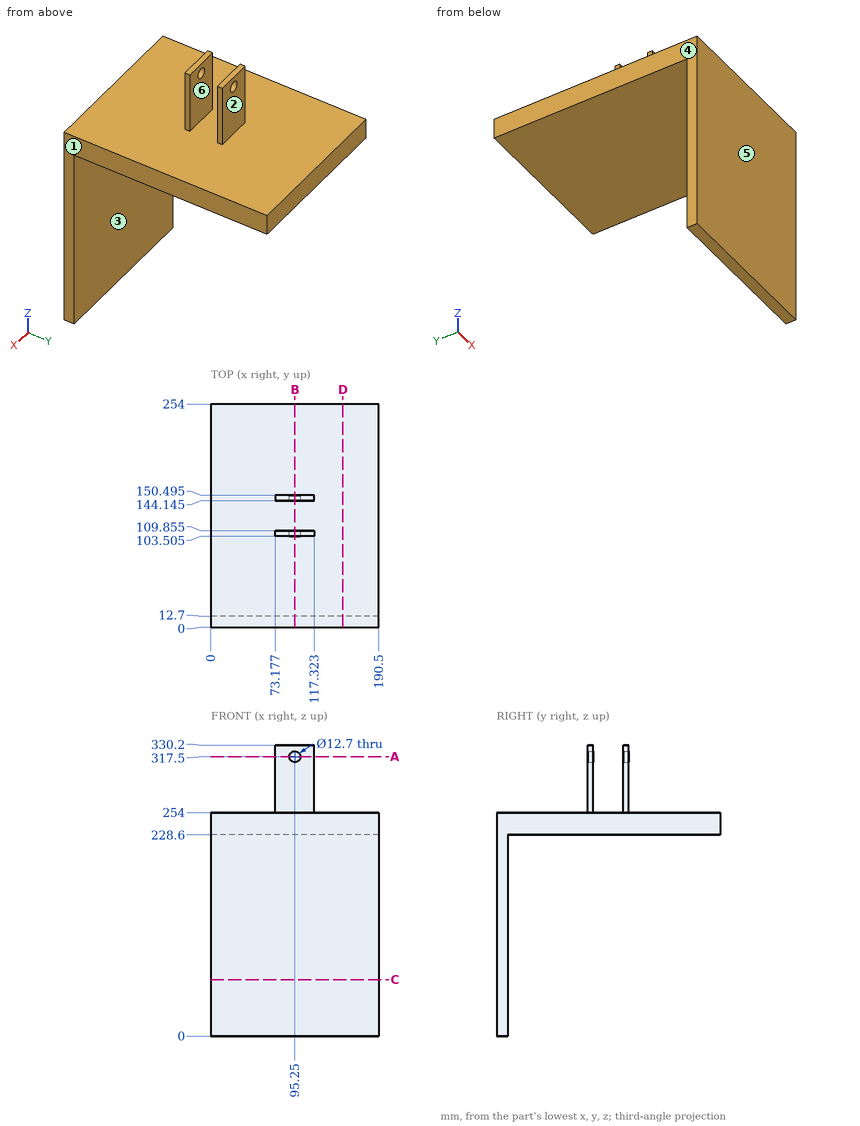
Study the drawing (mm; zero at the part's minimum x, y, z) and answer. A direction names the side the tool comes from. Give positions to 0.01 mm unless a question says otherwise; leave off trailing zeros. Order: outer loops, then holes, each group sorted by start corner. A loop starts at its lowest first (then second) coordinate and runs counter-clockwise, first axis right, second up. Notation, with made-up numbers: (32, 63.5) - (85, 63.5) arc R16 ccw to (85, 77.5) - close; hole circle Ø10 at (-37, -33.75). An arc over 180 degrees is marked (long way). Answer in a Markdown table with one row per item. Add a question column.
Q1. The part is cut by section B-B (x = 95.25). Give the number of separate pieces and of enclosed holes in the cut face, then the cut area to 3 significant figures.
Q2. The part is cut by section D-D (x = 150). Determine the outline of the cut face in (y, z).
Q3. Which of the six approach directions +Z, -Z, +X, -X, +Y, -Y give full straight-line access (tool end or side, diameter ignored) to the marked faces 1, 2 and 3?
Q4. Given P1, Ø8, axis at x = 62, z = 162.5, coming from the +Y side; P2, Ø7, axis at y = 148, z = 281, coming from the -X side; P3, Ø2, axis at x = 31.5, y = 194, coming from the -Z side, each flat-ended and moving along its own axis, determine where each tip first touches the part or whether it passes through.
Q5. The part is cut by section C-C (z = 64). Determine the outline of the cut face in (x, y).
Q6. For a pull along Y with two mould halves and no side action, classify the marked faces 4, 5 and 6 as released by +Y, released by -Y, zero draft, split by the parting line, or undercut.
Q7. The part is cut by section A-A (z = 317.5). Determine the outline of the cut face in (x, y) (1 decimal), then the cut area to 3 significant figures.
Q8. Find the intervals of material crossed by line 1 along Z through (x, y) = (95.25, 107.25); line 2 along Y through (x, z) = (113.5, 302.5) (1 decimal); line 3 along Y through (x, z) = (162, 89), in increasing order. Write a range as [from, to].
Determined:
| question | item | result |
|---|---|---|
| 1 | separate pieces | 3 |
| 1 | enclosed holes | 0 |
| 1 | area | 10,200 mm² |
| 2 | outline | (0, 0) - (12.7, 0) - (12.7, 228.6) - (254, 228.6) - (254, 254) - (0, 254) - close |
| 3 | face 1 | +Z, -Z, +X, +Y, -Y |
| 3 | face 2 | +Z, +X, -X, +Y |
| 3 | face 3 | -Z, +X, -X, +Y |
| 4 | P1 | stops at y = 12.7 |
| 4 | P2 | stops at x = 73.18 |
| 4 | P3 | stops at z = 228.6 |
| 5 | outline | (0, 0) - (190.5, 0) - (190.5, 12.7) - (0, 12.7) - close |
| 6 | face 4 | zero draft |
| 6 | face 5 | released by -Y |
| 6 | face 6 | undercut |
| 7 | outline | (73.2, 103.5) - (88.9, 103.5) - (88.9, 109.9) - (73.2, 109.9) - close; (73.2, 144.1) - (88.9, 144.1) - (88.9, 150.5) - (73.2, 150.5) - close; (101.6, 103.5) - (117.3, 103.5) - (117.3, 109.9) - (101.6, 109.9) - close; (101.6, 144.1) - (117.3, 144.1) - (117.3, 150.5) - (101.6, 150.5) - close |
| 7 | area | 399 mm² |
| 8 | line 1 | z = [228.6, 311.15], [323.85, 330.2] |
| 8 | line 2 | y = [103.5, 109.9], [144.1, 150.5] |
| 8 | line 3 | y = [0, 12.7] |
